Could you check a few things on this model? Use its own coordinates, in mm. A direction names the side the tool comes from. Give positions to 0.01 mm unless a question says otherwise; leave off trailing zeros. Loops run counter-clockwise (first coordinate to the right, second up) from the corner with the lowest first, then second, coordinate; pieces in that order, holes last. Notation, with made-up numbers: (-37.75, -8) -> (7.25, -8) arc R27 ccw to (7.25, 11) -> close; hole circle Ø10 at (20.5, 68). An arc over 180 degrees is marked (long way). Write item = value, one per line. Start each with the question number.
1) If we mould it in two halves opening along Z, with no side actions, what happens to faces 3 (the face through (42.85, -12.52, 0.33)), 4 (the face through (7, -16.331, -30)), 5 (the face through (33.381, -12.522, 19.693))? For each: +Z half, -Z half, draft (parallel to the pull), parting line (faces both ways), or undercut.
2) I need wall thicknesses on probe 1 along X at (y, z) = (-10, 5.5); probe 2 along Y at (x, z) = (29.5, -8); probe 3 along X at (y, z) = (-21, 3.5). Which ranges of each line are inside material? Lowest first, please. Write a range as from..to.
3) On a 3-axis mill with a long thin cutter (end or side, diameter ignored), from which of +Z, -Z, +X, -X, +Y, -Y can I reach the whole of each face in a straight line? I mean faces 1 (the face through (15, -27, -8.512)), 2 (the face through (19, 0, -2)). Say none if no direction works.
4) I want a section at B-B (x = -1). List the corners of the cut face in (y, z) for me, and give its area (3 significant figures).
5) I want a section at C-C (y = -50). List the corners of the cut face in (x, z) for me.
6) I want a section at A-A (y = -9.5). List the corners of the cut face in (x, z) for me.
7) I want a section at D-D (z = -26). List the corners of the cut face in (x, y) for me.
8) I'm going to push flat-ended pins straight in: pin 1 Ø2 at (x, y) = (16, -16) entering from +Z; pin 2 Ø3 at (y, z) = (-38, -4.5) entering from +X; pin 3 Ø10 at (x, y) = (23.5, -17.5) entering from -Z. Where does each tip first touch, or does it pass through?
from build123d import *

# Parameters (mm, degrees)
F0_R     = 7.6083781551
F1_DEPTH = 25.4
F2_DEPTH = 16.33147
F3_DEPTH = 54.06381


with BuildPart() as f1:
    # F0 (on Front) → F1 (new body)
    with BuildSketch(Plane.XZ):
        with BuildLine():
            ThreePointArc((13.9462792399, -27.3820497182), (24.5288614061, -16.9645417548), (28.40983312, -2.6308898814))
            ThreePointArc((28.40983312, -2.6308898814), (24.3839357983, 11.9479404177), (13.4472466105, 22.394900346))
            ThreePointArc((13.4472466105, 22.394900346), (-27.5508361213, 4.3023667074), (0, -31.0407230014))
            Line((0, -31.0407230014), (13.9462792399, -27.3820497182))
        make_face()
        with BuildLine():
            ThreePointArc((-13.0795865189, 0), (0, 10.7106679389), (13.0795865189, 0))
            Line((13.0795865189, 0), (18.5709875077, 0))
            Line((18.5709875077, 0), (18.5709875077, -8.5117025301))
            Line((18.5709875077, -8.5117025301), (11.9755253606, -8.5117025301))
            ThreePointArc((11.9755253606, -8.5117025301), (0, -15.9724477017), (-11.9755253606, -8.5117025301))
            Line((-11.9755253606, -8.5117025301), (-17.9519541562, -8.5117025301))
            Line((-17.9519541562, -8.5117025301), (-17.9519541562, 0))
            Line((-17.9519541562, 0), (-13.0795865189, 0))
        make_face(mode=Mode.SUBTRACT)
        with BuildLine():
            ThreePointArc((13.4472466105, 22.394900346), (24.3839357983, 11.9479404177), (28.40983312, -2.6308898814))
            ThreePointArc((28.40983312, -2.6308898814), (24.5288614061, -16.9645417548), (13.9462792399, -27.3820497182))
            Line((13.9462792399, -27.3820497182), (54.8214644814, -16.6588349012))
            ThreePointArc((54.8214644814, -16.6588349012), (33.2605864945, -1.0486865195), (52.764098421, 17.0665340036))
            Line((52.764098421, 17.0665340036), (13.4472466105, 22.394900346))
        make_face()
        with BuildLine():
            ThreePointArc((67.6737267911, 0), (63.4213470707, 11.3309708435), (52.764098421, 17.0665340036))
            ThreePointArc((52.764098421, 17.0665340036), (33.2605864945, -1.0486865195), (54.8214644814, -16.6588349012))
            ThreePointArc((54.8214644814, -16.6588349012), (64.0872268937, -10.5201880537), (67.6737267911, 0))
        make_face()
        with Locations((50.4511781037, 0)):
            Circle(F0_R, mode=Mode.SUBTRACT)
        with BuildLine():
            ThreePointArc((-11.9755253606, -8.5117025301), (-13.2307190966, -4.3470592374), (-13.0795865189, 0))
            Line((-13.0795865189, 0), (-17.9519541562, 0))
            Line((-17.9519541562, 0), (-17.9519541562, -8.5117025301))
            Line((-17.9519541562, -8.5117025301), (-11.9755253606, -8.5117025301))
        make_face()
    extrude(amount=F1_DEPTH)

    # F0 (on Front) → F2 (join)
    with BuildSketch(Plane.XZ):
        with BuildLine():
            ThreePointArc((13.9462792399, -27.3820497182), (24.5288614061, -16.9645417548), (28.40983312, -2.6308898814))
            ThreePointArc((28.40983312, -2.6308898814), (24.3839357983, 11.9479404177), (13.4472466105, 22.394900346))
            ThreePointArc((13.4472466105, 22.394900346), (-27.5508361213, 4.3023667074), (0, -31.0407230014))
            Line((0, -31.0407230014), (13.9462792399, -27.3820497182))
        make_face()
        with BuildLine():
            ThreePointArc((-13.0795865189, 0), (0, 10.7106679389), (13.0795865189, 0))
            Line((13.0795865189, 0), (18.5709875077, 0))
            Line((18.5709875077, 0), (18.5709875077, -8.5117025301))
            Line((18.5709875077, -8.5117025301), (11.9755253606, -8.5117025301))
            ThreePointArc((11.9755253606, -8.5117025301), (0, -15.9724477017), (-11.9755253606, -8.5117025301))
            Line((-11.9755253606, -8.5117025301), (-17.9519541562, -8.5117025301))
            Line((-17.9519541562, -8.5117025301), (-17.9519541562, 0))
            Line((-17.9519541562, 0), (-13.0795865189, 0))
        make_face(mode=Mode.SUBTRACT)
        with BuildLine():
            ThreePointArc((13.4472466105, 22.394900346), (24.3839357983, 11.9479404177), (28.40983312, -2.6308898814))
            ThreePointArc((28.40983312, -2.6308898814), (24.5288614061, -16.9645417548), (13.9462792399, -27.3820497182))
            Line((13.9462792399, -27.3820497182), (54.8214644814, -16.6588349012))
            ThreePointArc((54.8214644814, -16.6588349012), (33.2605864945, -1.0486865195), (52.764098421, 17.0665340036))
            Line((52.764098421, 17.0665340036), (13.4472466105, 22.394900346))
        make_face()
        with BuildLine():
            ThreePointArc((0, -31.0407230014), (7.2091017962, -30.1108365553), (13.9462792399, -27.3820497182))
            Line((13.9462792399, -27.3820497182), (0, -31.0407230014))
        make_face()
        with BuildLine():
            ThreePointArc((67.6737267911, 0), (63.4213470707, 11.3309708435), (52.764098421, 17.0665340036))
            ThreePointArc((52.764098421, 17.0665340036), (33.2605864945, -1.0486865195), (54.8214644814, -16.6588349012))
            ThreePointArc((54.8214644814, -16.6588349012), (64.0872268937, -10.5201880537), (67.6737267911, 0))
        make_face()
        with Locations((50.4511781037, 0)):
            Circle(F0_R, mode=Mode.SUBTRACT)
    extrude(amount=F2_DEPTH)

    # F0 (on Front) → F3 (join)
    with BuildSketch(Plane.XZ):
        with BuildLine():
            ThreePointArc((13.9462792399, -27.3820497182), (24.5288614061, -16.9645417548), (28.40983312, -2.6308898814))
            ThreePointArc((28.40983312, -2.6308898814), (24.3839357983, 11.9479404177), (13.4472466105, 22.394900346))
            ThreePointArc((13.4472466105, 22.394900346), (-27.5508361213, 4.3023667074), (0, -31.0407230014))
            Line((0, -31.0407230014), (13.9462792399, -27.3820497182))
        make_face()
        with BuildLine():
            ThreePointArc((-13.0795865189, 0), (0, 10.7106679389), (13.0795865189, 0))
            Line((13.0795865189, 0), (18.5709875077, 0))
            Line((18.5709875077, 0), (18.5709875077, -8.5117025301))
            Line((18.5709875077, -8.5117025301), (11.9755253606, -8.5117025301))
            ThreePointArc((11.9755253606, -8.5117025301), (0, -15.9724477017), (-11.9755253606, -8.5117025301))
            Line((-11.9755253606, -8.5117025301), (-17.9519541562, -8.5117025301))
            Line((-17.9519541562, -8.5117025301), (-17.9519541562, 0))
            Line((-17.9519541562, 0), (-13.0795865189, 0))
        make_face(mode=Mode.SUBTRACT)
        with BuildLine():
            ThreePointArc((-11.9755253606, -8.5117025301), (-13.2307190966, -4.3470592374), (-13.0795865189, 0))
            Line((-13.0795865189, 0), (-17.9519541562, 0))
            Line((-17.9519541562, 0), (-17.9519541562, -8.5117025301))
            Line((-17.9519541562, -8.5117025301), (-11.9755253606, -8.5117025301))
        make_face()
    extrude(amount=F3_DEPTH)


solid = f1.part
Answer list:
q1.face_3 = undercut
q1.face_4 = draft
q1.face_5 = +Z half
q2.probe_1 = -27.22..-10.58, 10.58..45.19, 55.71..66.77
q2.probe_2 = -25.4..0
q2.probe_3 = -27.74..-11.85, 11.85..43.7, 57.21..67.31
q3.face_1 = +Y, -Y
q3.face_2 = +Z, -Z, +X, -X, +Y
q4.outline = (-54.06, -31.02) -> (0, -31.02) -> (0, -15.93) -> (-54.06, -15.93) -> close; (-54.06, 10.67) -> (0, 10.67) -> (0, 25.76) -> (-54.06, 25.76) -> close
q4.area = 1,630 mm^2
q5.outline = (0, -31.04) -> (13.95, -27.38) arc R28.41 ccw (long way) to start; hole (11.98, -8.51) -> (18.57, -8.51) -> (18.57, 0) -> (13.08, 0) arc R13.34 ccw (long way) to start
q6.outline = (13.45, 22.39) arc R28.41 ccw (long way) to (13.95, -27.38) -> (54.82, -16.66) arc R17.22 ccw to (52.76, 17.07) -> close; hole (11.98, -8.51) -> (18.57, -8.51) -> (18.57, 0) -> (13.08, 0) arc R13.34 ccw (long way) to start; hole circle Ø15.22 at (50.45, 0)
q7.outline = (-16.16, -54.06) -> (16.16, -54.06) -> (16.16, -25.4) -> (19.21, -25.4) -> (19.21, 0) -> (-16.16, 0) -> close
q8.pin_1 = 22.18
q8.pin_2 = 28.41
q8.pin_3 = -26.19
